Check sheet for the drawn part. Datum: minimum x, y, z corner. Units: mm. Coordinates: 2 decimals unless noted, no trailing zeros. Write each loop counter-clockwise with the first axis right and the second up, starting at its lowest first coordinate (ties: lowest second). Pieces come first, ordered by that corner, then holes. Notation, with made-up numbers: M 27,24 L 32,24 A29 cw 32,51 Z; hole C 57,6 d5. An arc over 180 degrees is marked long. Answer as CSV lines item,"result".
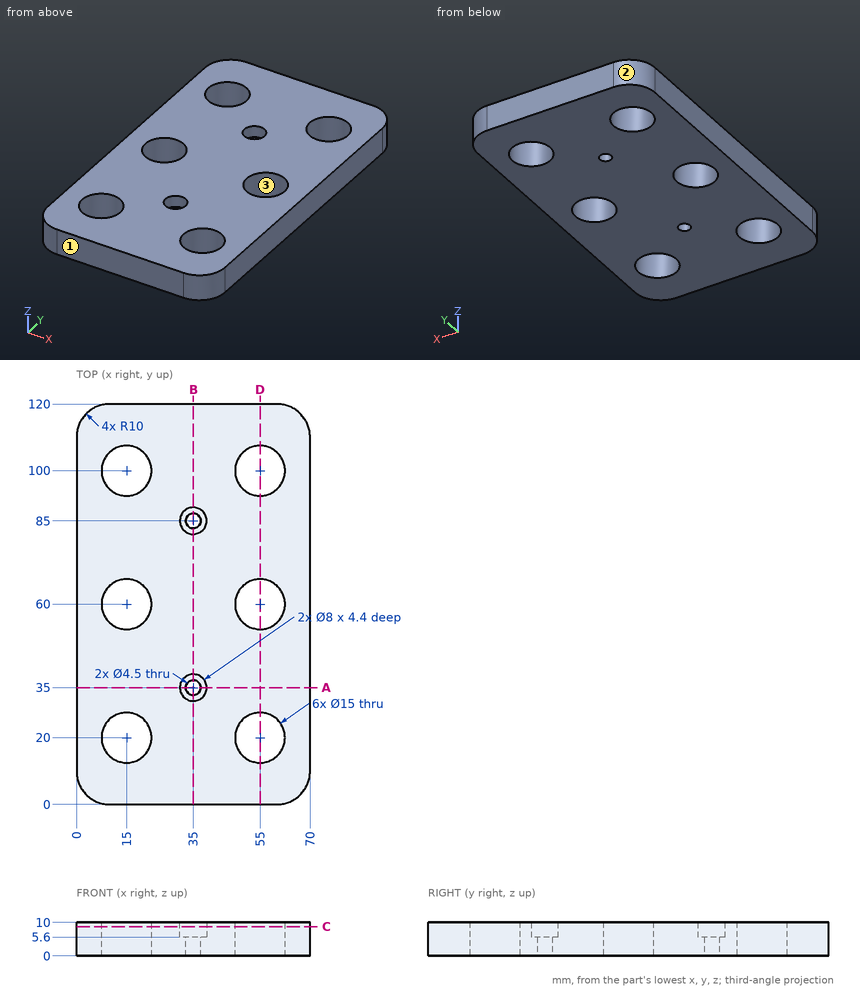
1) Section check D-D, the plane x = 55. Record the boundary of the cut face in (y, z).
Answer key:
outline,"M 0,0 L 12.5,0 L 12.5,10 L 0,10 Z; M 27.5,0 L 52.5,0 L 52.5,10 L 27.5,10 Z; M 67.5,0 L 92.5,0 L 92.5,10 L 67.5,10 Z; M 107.5,0 L 120,0 L 120,10 L 107.5,10 Z"
2) Mould release check, pull along X, two halves, no side actions. Record for the marked faces 1, 2 and 3: pulls with the +X half, pulls with the -X half, needs draft (parallel to the pull), parting line crosses it, or undercut.
Answer key:
face 1,"needs draft"
face 2,"pulls with the -X half"
face 3,"undercut"
3) Section check C-C, the plane z = 8.75. Give the number of separate pieces and of enclosed holes in the cut face, plus the area to 3 significant figures.
Answer key:
separate pieces,"1"
enclosed holes,"8"
area,"7,150 mm2"
4) Thickness scan on line 1 along Y through (x, z) = (15, 5.75); line 2 along Y through (x, z) = (35, 8.3); line 3 along X through (y, z) = (20.5, 4.5). Record the ranges inside material, lowest first.
Answer key:
line 1,"y = 0 to 12.5, 27.5 to 52.5, 67.5 to 92.5, 107.5 to 120"
line 2,"y = 0 to 31, 39 to 81, 89 to 120"
line 3,"x = 0 to 7.52, 22.48 to 47.52, 62.48 to 70"
5) Section check A-A, the plane y = 35. Record the boundary of the cut face in (x, z).
Answer key:
outline,"M 0,0 L 32.75,0 L 32.75,5.6 L 31,5.6 L 31,10 L 0,10 Z; M 37.25,0 L 70,0 L 70,10 L 39,10 L 39,5.6 L 37.25,5.6 Z"
6) Depth check by flat-ended pin: P1, Ø2.5, axis at x = 36, y = 84, coming from the +Z side. Enter the tip coordinate at first touch or a pass-through.
Answer key:
P1,"stops at z = 5.6"
7) Section check B-B, the plane x = 35. Record the boundary of the cut face in (y, z), plus the area to 3 significant figures.
Answer key:
outline,"M 0,0 L 32.75,0 L 32.75,5.6 L 31,5.6 L 31,10 L 0,10 Z; M 37.25,0 L 82.75,0 L 82.75,5.6 L 81,5.6 L 81,10 L 39,10 L 39,5.6 L 37.25,5.6 Z; M 87.25,0 L 120,0 L 120,10 L 89,10 L 89,5.6 L 87.25,5.6 Z"
area,"1,080 mm2"
